```python
from build123d import *

# Parameters (mm, degrees)
BOSS_EXTRUDE1_DEPTH      = 7
FILLET1_R                = 4
BOSS_EXTRUDE2_DEPTH      = 3
BOSS_EXTRUDE2_DEPTH_BACK = 9.99999997
SKETCH2_R                = 3.75
CUT_EXTRUDE1_DEPTH       = 38.480069693


with BuildPart() as part:
    # Sketch1 → Boss-Extrude1 (new body)
    with BuildSketch(Plane.XY):
        Polygon((4, 25.4), (4, 34.925), (-4, 34.925), (-4, 25.4), (-4, -25.4), (4, -25.4), align=None)
    extrude(amount=BOSS_EXTRUDE1_DEPTH)

    # Fillet1
    fillet1_edges = [part.edges().sort_by_distance(p)[0] for p in [
        (-4, -25.4, 3.5),
        (4, -25.4, 3.5),
        (4, 34.925, 3.5),
        (-4, 34.925, 3.5),
    ]]
    fillet(fillet1_edges, radius=FILLET1_R - 0.0001)  # a hair under: the kernel refuses the full size

    # Sketch2 → Boss-Extrude2 (add, two sides: drawn at the far end of the back side and taken through both)
    with BuildSketch(Plane.XY.offset(7).offset(-BOSS_EXTRUDE2_DEPTH_BACK)):
        with Locations((0, 20.32)):
            Circle(SKETCH2_R)
    extrude(amount=BOSS_EXTRUDE2_DEPTH + BOSS_EXTRUDE2_DEPTH_BACK)

    # Sketch3 → Cut-Extrude1 (cut, through all)
    with BuildSketch(Plane(origin=(0, 0, -2.99999997), x_dir=(-1, 0, 0), z_dir=(0, 0, -1))):
        with BuildLine():
            Line((-0.889, 21.1455), (-0.889, 22.7965))
            ThreePointArc((-0.889, 22.7965), (0, 22.953207345), (0.889, 22.7965))
            Line((0.889, 22.7965), (0.889, 21.1455))
            Line((0.889, 21.1455), (2.54, 21.1455))
            ThreePointArc((2.54, 21.1455), (2.674528493, 20.32), (2.54, 19.4945))
            Line((2.54, 19.4945), (0.889, 19.4945))
            Line((0.889, 19.4945), (0.889, 17.8435))
            ThreePointArc((0.889, 17.8435), (0, 17.686792655), (-0.889, 17.8435))
            Line((-0.889, 17.8435), (-0.889, 19.4945))
            Line((-0.889, 19.4945), (-2.54, 19.4945))
            ThreePointArc((-2.54, 19.4945), (-2.674528493, 20.32), (-2.54, 21.1455))
            Line((-2.54, 21.1455), (-0.889, 21.1455))
        make_face()
    extrude(amount=-CUT_EXTRUDE1_DEPTH, mode=Mode.SUBTRACT)


solid = part.part
```
Check sheet for the modelled part. Datum: model origin and axes. Units: mm. A direction names the side the tool comes from. Give positions to 0.01 mm unless a question says otherwise; leave off trailing zeros. Write each loop counter-clockwise with the first axis right and the second up, starting at its lowest first coordinate (ties: lowest second). Pieces come first, ordered by that corner, then holes. Notation, with made-up numbers: (4, -16.75) - (18, -16.75) arc R10 ccw to (18, -12.75) - close; hole circle Ø11 at (18.5, -5.5). An arc over 180 degrees is marked (long way). Answer as a JSON object with one key per item and string values. Group by question number.
1) Thickness scan on probe 1 along Z at (x, y) = (-2, -13.5); probe 2 along X at (y, z) = (-21.5, 5); probe 3 along Y at (x, z) = (-1.5, 5). Record the ranges inside material, lowest first. Write a range as from..to.
2) Sectioned sample at B-B (y = 20.32). Record the cut outline in (x, z), then the cut area to 3 significant figures.
3) Depth check by flat-ended pin: P1, Ø3, axis at x = -2.5, y = 5.5, coming from the +Z side; P2, Ø4, axis at x = 0, y = 7, coming from the -Z side; P3, Ø1.8, axis at x = -2, z = 2.5, coming from the +Y side. Enter the tip coordinate at first touch or a pass-through.
4) Release check for a two-part mould opening along X. For faces 1 (the face through (0, 5, 0)), 2 (the face through (2, 19.494, 3)), 3 (the face through (-2.8, 33.78, 3.55)) record: pulls with the +X half, pulls with the -X half, needs draft (parallel to the pull), parting line crosses it, or undercut.
5) Sectioned sample at C-C (z = 9.25). Record the cut outline in (x, y).
6) Access from +Z, -Z, +X, -X, +Y, -Y to the whole of each face (thin tool, end or side, straight path). Record for faces 4 (the face through (-0.488, 24.038, -1.521)), 5 (the face through (0.889, 19, 3)), 6 (the face through (4, 4, 3)).
7) Sectioned sample at D-D (y = 6). Record the cut outline in (x, z), then the cut area to 3 significant figures.
Geometry results:
{
 "1": {"probe 1": "z = 0..7", "probe 2": "x = -4..4", "probe 3": "y = -25.11..19.49, 21.15..34.63"},
 "2": {"outline": "(-4, 0) - (-3.75, 0) - (-3.75, -3) - (-2.67, -3) - (-2.67, 10) - (-3.75, 10) - (-3.75, 7) - (-4, 7) - close; (2.67, -3) - (3.75, -3) - (3.75, 0) - (4, 0) - (4, 7) - (3.75, 7) - (3.75, 10) - (2.67, 10) - close", "area": "31.5 mm^2"},
 "3": {"P1": "stops at z = 7", "P2": "stops at z = 0", "P3": "stops at y = 34.77"},
 "4": {"face 1": "needs draft", "face 2": "undercut", "face 3": "pulls with the -X half"},
 "5": {"outline": "circle Ø7.5 at (0, 20.32); hole (-2.54, 19.49) - (-0.89, 19.49) - (-0.89, 17.84) arc R2.6 ccw to (0.89, 17.84) - (0.89, 19.49) - (2.54, 19.49) arc R2.6 ccw to (2.54, 21.15) - (0.89, 21.15) - (0.89, 22.8) arc R2.6 ccw to (-0.89, 22.8) - (-0.89, 21.15) - (-2.54, 21.15) arc R2.6 ccw to start"},
 "6": {"face 4": "-Z", "face 5": "+Z, -Z", "face 6": "+Z, -Z, +X, +Y, -Y"},
 "7": {"outline": "(-4, 0) - (4, 0) - (4, 7) - (-4, 7) - close", "area": "56.0 mm^2"}
}
